Check sheet for the modelled part. Datum: model origin and axes. Units: mm. Give positions to 0.01 mm unless a question says otherwise; leave off trailing zeros. Order: outer loops, then holes, each group sorted by start corner. A loop starts at its lowest first (then second) coordinate and runs counter-clockwise, first axis right, second up.
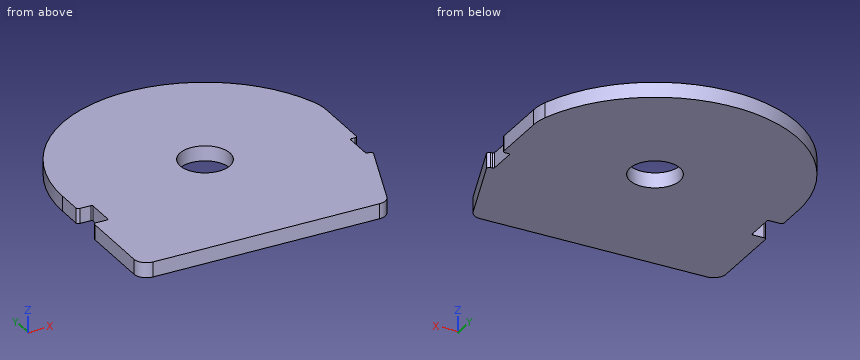
Autodesk Inventor part; units mm, degrees
ref_plane "YZ Plane" through (0, 0, 0) normal (1, 0, 0) x (0, 1, 0)
ref_plane "XZ Plane" through (0, 0, 0) normal (0, 1, 0) x (-1, 0, 0)
ref_plane "XY Plane" through (0, 0, 0) normal (0, 0, 1) x (1, 0, 0)
sketch "Sketch1" plane through (0, 0, 0) normal (0, 0, 1) x (1, 0, 0)
  circle A0 centre (0, 0) radius 10
  line L0 (-57, -58) -> (42, -58)
  line L1 (42, -58) -> (54.739, -23)
  line L2 (54.739, -23) -> (52, -23)
  line L3 (52, -23) -> (52, -11)
  line L4 (52, -11) -> (55, -11)
  line L5 (55, -11) -> (55, 12)
  line L6 (-57, -58) -> (-57, -23)
  line L7 (-57, -23) -> (-51, -23)
  line L8 (-51, -23) -> (-51, -11)
  line L9 (-51, -11) -> (-57, -11)
  line L10 (-57, -11) -> (-57, 0)
  arc A1 (53.9189, 18.4865) -> (-57, 0) centre (0, 0) ccw
  arc A2 (55, 12) -> (53.9189, 18.4865) centre (35, 12) ccw
  dimension "d0" = 20
  dimension "d1" = 57
  dimension "d2" = 20
  dimension "d3" = 99
  dimension "d4" = 6
  dimension "d5" = 110
  dimension "d6" = 3
  dimension "d7" = 12
  dimension "d8" = 58
  dimension "d9" = 12
  dimension "d10" = 55
  dimension "d11" = 47
extrude "Extrusion1" add sketch "Sketch1" along normal blind 6
fillet "Fillet1" radius 0.5 4 edges at (52, -23, 3) (52, -11, 3) (-51, -11, 3) (-51, -23, 3)
fillet "Fillet2" radius 1 4 edges at (-57, -11, 3) (-57, -23, 3) (55, -11, 3) (54.739, -23, 3)
fillet "Fillet3" radius 5 2 edges at (42, -58, 3) (-57, -58, 3)
properties part number "NPT Flange Inner"
(1) Cross-section at C-C on y = -3.5. Enter the section's corners in (x, z).
Response values:
outline: (-57, 0) - (-9.37, 0) - (-9.37, 6) - (-57, 6) - close; (9.37, 0) - (55, 0) - (55, 6) - (9.37, 6) - close
(2) Cross-section at B-B on z = 2.75. Enter the section's corners in (x, y).
Response values:
outline: (-57, -53) arc R5 ccw to (-52, -58) - (38.5, -58) arc R5 ccw to (43.2, -54.71) - (54.25, -24.34) arc R1 ccw to (53.31, -23) - (52.5, -23) arc R0.5 cw to (52, -22.5) - (52, -11.5) arc R0.5 cw to (52.5, -11) - (54, -11) arc R1 ccw to (55, -10) - (55, 12) arc R20 ccw to (53.92, 18.49) arc R57 ccw to (-57, 0) - (-57, -10) arc R1 ccw to (-56, -11) - (-51.5, -11) arc R0.5 cw to (-51, -11.5) - (-51, -22.5) arc R0.5 cw to (-51.5, -23) - (-56, -23) arc R1 ccw to (-57, -24) - close; hole circle Ø20 at (0, 0)
(3) Material ranges on L1, parallel to Y at x = 0, z = 1.3; L2, parallel to X at y = -3.5, z = 1.65; L3, parallel to X at y = -19, z = 2.25, recorded low to high.
Response values:
L1: y = -58 to -10, 10 to 57
L2: x = -57 to -9.37, 9.37 to 55
L3: x = -51 to 52
(4) Cross-section at A-A on x = 0. Enter the section's corners in (y, z), then the cut area to 3 significant figures.
Response values:
outline: (-58, 0) - (-10, 0) - (-10, 6) - (-58, 6) - close; (10, 0) - (57, 0) - (57, 6) - (10, 6) - close
area: 570 mm2
(5) Gauge pin test, flat ends, axial feed: pin 1 Ø1.8 at (y, z) = (-18.5, 2.5) entering from -X; pin 2 Ø1.3 at (x, z) = (-53.5, 3.5) entering from +Y; pin 3 Ø4 at (x, y) = (33.5, 38.5) entering from -Z. Record the tip position at first contact, or that the pin passes through.
Response values:
pin 1: stops at x = -51
pin 2: stops at y = 21.35
pin 3: stops at z = 0
(6) Cross-section at D-D on y = -15. Enter the section's corners in (x, z), then the cut area to 3 significant figures.
Response values:
outline: (-51, 0) - (52, 0) - (52, 6) - (-51, 6) - close
area: 618 mm2
